from build123d import *

# Parameters (mm, degrees)
F0_R     = 2.55
F1_DEPTH = 10
F2_W     = 20.1
F2_H     = 5
F3_DEPTH = 50.001
F5_DEPTH = 50
F6_DEPTH = 10
F7_DEPTH = 4.5
F8_DEPTH = 1
F9_R     = 3
F10_SIZE = 2.2
F11_SIZE = 1


# Not quite as in the source:
# - a feature names something its author has since deleted; it is built from what else it names


with BuildPart() as f1:
    # F0 (on Top) → F1 (new body)
    with BuildSketch(Plane.XY):
        with BuildLine():
            Line((-8.8436374201, 26.9644671741), (-15, 10.05))
            Line((-15, 10.05), (-15, -10.05))
            Line((-15, -10.05), (-8.8436374201, -26.9644671741))
            ThreePointArc((-8.8436374201, -26.9644671741), (-2.7616213035, -32.7425446245), (5.5147415904, -31.3718089411))
            Line((5.5147415904, -31.3718089411), (35, -10.05))
            Line((35, -10.05), (35, 10.05))
            Line((35, 10.05), (5.5147415904, 31.3718089411))
            ThreePointArc((5.5147415904, 31.3718089411), (-2.7616213035, 32.7425446245), (-8.8436374201, 26.9644671741))
        make_face()
        with Locations((0, -24)):
            Circle(F0_R, mode=Mode.SUBTRACT)
        with Locations((-7, 0)):
            Circle(F0_R, mode=Mode.SUBTRACT)
        with Locations((0, 24)):
            Circle(F0_R, mode=Mode.SUBTRACT)
        with Locations((27, 0)):
            Circle(F0_R, mode=Mode.SUBTRACT)
    extrude(amount=F1_DEPTH)

    # F2 (on face) → F3 (cut, through all)
    with BuildSketch(Plane(origin=(-15, 0, 0), x_dir=(0, -1, 0), z_dir=(-1, 0, 0))):
        with Locations((0, 2.5)):
            Rectangle(F2_W, F2_H)
    extrude(amount=-F3_DEPTH, mode=Mode.SUBTRACT)

    # F4 (on face) → F5 (join, through all)
    with BuildSketch(Plane(origin=(-15, 0, 0), x_dir=(0, -1, 0), z_dir=(-1, 0, 0))):
        Polygon((3.05, 3.545), (4.5, 5), (-4.5, 5), (-3.05, 3.545), align=None)
    extrude(amount=-F5_DEPTH)

    # F0 (on Top) → F6 (cut, through all)
    with BuildSketch(Plane.XY):
        with Locations((-7, 0)):
            Circle(F0_R)
        with Locations((27, 0)):
            Circle(F0_R)
    extrude(amount=F6_DEPTH, mode=Mode.SUBTRACT)

    # F7 (add): a face of the model
    f7_faces = [f1.faces().sort_by_distance(p)[0] for p in [
        (5.7473624585, -18.668206632, 0),
    ]]
    extrude(f7_faces, amount=F7_DEPTH)

    # F8 (cut): a face of the model
    f8_faces = [f1.faces().sort_by_distance(p)[0] for p in [
        (5.7473624585, 18.668206632, 0),
    ]]
    extrude(f8_faces, amount=-F8_DEPTH, mode=Mode.SUBTRACT)

    # F9
    f9_edges = [f1.edges().sort_by_distance(p)[0] for p in [
        (-11.921819, 18.507234, 10),
        (-15, 0, 10),
        (-11.921819, -18.507234, 10),
        (35, 0, 10),
        (-2.761621, 32.742545, 10),
        (-2.761621, -32.742545, 10),
        (20.257371, -20.710904, 10),
        (20.257371, 20.710904, 10),
    ]]
    fillet(f9_edges, radius=F9_R)

    # F10
    f10_edges = [f1.edges().sort_by_distance(p)[0] for p in [
        (-2.55, -24, 10),
        (-9.55, 0, 10),
        (-2.55, 24, 10),
        (24.45, 0, 10),
    ]]
    chamfer(f10_edges, length=F10_SIZE)

    # F11
    f11_edges = [f1.edges().sort_by_distance(p)[0] for p in [
        (35, 10.05, 3),
        (5.514742, -31.371809, 1.25),
        (35, -10.05, 0.25),
    ]]
    chamfer(f11_edges, length=F11_SIZE)


solid = f1.part
Could you check a few things on this model? Use its own coordinates, in mm. A direction names the side the tool comes from. Coordinates: 2 decimals unless noted, no trailing zeros. Order: outer loops, then holes, each group sorted by start corner. A loop starts at its lowest first (then second) coordinate and runs counter-clockwise, first axis right, second up. Notation, with made-up numbers: (64, 8) - (88, 8) arc R12 cw to (88, 14) - close; hole circle Ø5 at (83, -24.5). An arc over 180 degrees is marked (long way). Answer in a Markdown table with one row per item. Add a question column.
(1) On a 3-axis mill with a long thin cutter (end or side, diameter ignored), from which of +Z, -Z, +X, -X, +Y, -Y can I reach the whole of each face in a straight line? I mean faces 5 (the face through (10, 0, 3.545)), 6 (the face through (10, 0, 10)), 7 (the face through (4, 19, 1)). Say none if no direction works.
(2) I need wall thicknesses on L1, parallel to X at y = 0, z = 5.6; L2, parallel to Y at x = 0, z = -0.5; L3, parallel to Y at x = 13, z = 4. Which ranges of each line are inside material? Lowest first, please.
(3) If we section it at B-B, the plane y = -6.5: Please give me the cut outline in (x, z), then the cut area to 3 significant figures.
(4) Will these pins go through, and if not, where does the flat tip stop? pin 1 (12 mm diameter, centred on x = 9, y = 25.5, fed in from -Z); pin 2 (1 mm diameter, centred on x = 19, z = 4.5, fed in from +Y); pin 3 (6 mm diameter, centred on x = -7, y = 0, fed in from -Z) (3 decimals).
(5) If we mould it in two halves opening along Y, with no side actions, what happens to faces 1 (the face through (1.18, -26.26, 1.56)), 2 (the face through (19.96, -19.87, 9.1)), 3 (the face through (10, 8, 5)), 4 (the face through (-11.12, 18.08, 9.14))? For each: released by +Y, released by -Y, zero draft, split by the parting line, or undercut.
(6) If we section it at C-C, the plane x = 0.5: State how many separate pieces and enclosed holes the cut face has, then the cut area to 3 significant figures.
(7) If we section it at A-A, the plane z = 2.5: Please give me the cut outline in (x, y), then the cut area to 3 significant figures.
Results are:
| question | item | result |
|---|---|---|
| 1 | face 5 | -Z, +X, -X |
| 1 | face 6 | +Z, +X, -X, +Y, -Y |
| 1 | face 7 | -Z, +X, -X, +Y |
| 2 | L1 | x = -15 to -9.55, -4.45 to 24.45, 29.55 to 35 |
| 2 | L2 | y = -33.16 to -26.55, -21.45 to -10.05 |
| 2 | L3 | y = -25.96 to -10.05, -3.5 to 3.5, 10.05 to 25.96 |
| 3 | outline | (-15, 5) - (35, 5) - (35, 7) arc R3 ccw to (32, 10) - (-12, 10) arc R3 ccw to (-15, 7) - close |
| 3 | area | 246 mm2 |
| 4 | pin 1 | stops at z = 1 |
| 4 | pin 2 | stops at y = 21.98 |
| 4 | pin 3 | stops at z = 3.545 |
| 5 | face 1 | undercut |
| 5 | face 2 | released by -Y |
| 5 | face 3 | undercut |
| 5 | face 4 | released by +Y |
| 6 | separate pieces | 3 |
| 6 | enclosed holes | 0 |
| 6 | area | 523 mm2 |
| 7 | outline | (-15, -10.05) - (-8.84, -26.96) arc R9.41 ccw to (5.51, -31.37) - (34.19, -10.64) - (34, -10.05) - close; (-15, 10.05) - (34, 10.05) - (34.19, 10.64) - (5.51, 31.37) arc R9.41 ccw to (-8.84, 26.96) - close; hole circle Ø5.1 at (0, -24); hole circle Ø5.1 at (0, 24) |
| 7 | area | 1,320 mm2 |
